from build123d import *

# Parameters (mm, degrees)
BOSS_EXTRUDE1_DEPTH      = 0.5
BOSS_EXTRUDE1_DEPTH_BACK = 38
SKETCH1_R                = 2
BOSS_EXTRUDE2_DEPTH      = 1
BOSS_EXTRUDE2_DEPTH_BACK = 0.2
FILLET1_R                = 1
SKETCH3_W                = 9.33031097
SKETCH3_H                = 7.737675748
BOSS_EXTRUDE3_DEPTH      = 0.5


with BuildPart() as part:
    # Sketch1 → Boss-Extrude1 (new, two sides: drawn at the far end of the back side and taken through both)
    with BuildSketch(Plane.XY.offset(-BOSS_EXTRUDE1_DEPTH_BACK)):
        with Locations((36.163012657, 38.866961635)):
            Circle(SKETCH1_R)
    extrude(amount=BOSS_EXTRUDE1_DEPTH + BOSS_EXTRUDE1_DEPTH_BACK)

    # Sketch2 → Boss-Extrude2 (add, two sides: drawn at the far end of the back side and taken through both)
    with BuildSketch(Plane.XY.offset(0.5).offset(-BOSS_EXTRUDE2_DEPTH_BACK)):
        with BuildLine():
            Line((36.163012657, 33.665102482), (42.084431795, 43.04323939))
            add(Edge.make_bspline(
                [(42.084431795, 43.04323939), (36.188063939, 40.196898594), (30.297901751, 43.04323939)],
                knots=[0, 0, 0, 1, 1, 1], degree=2))
            Line((30.297901751, 43.04323939), (36.163012657, 33.665102482))
        make_face()
    extrude(amount=BOSS_EXTRUDE2_DEPTH + BOSS_EXTRUDE2_DEPTH_BACK)

    # Fillet1
    fillet1_edges = [part.edges().sort_by_distance(p)[0] for p in [
        (33.230457204, 38.354170936, 1.5),
        (39.123722226, 38.354170936, 1.5),
        (36.189615356, 41.620068992, 1.5),
    ]]
    fillet(fillet1_edges, radius=FILLET1_R - 0.0001)  # a hair under: the kernel refuses the full size

    # Sketch3 → Boss-Extrude3 (add)
    with BuildSketch(Plane.XY.offset(-2.1)):
        with Locations((36.163012657, 38.866961635)):
            Rectangle(SKETCH3_W, SKETCH3_H)
    extrude(amount=-BOSS_EXTRUDE3_DEPTH)


solid = part.part
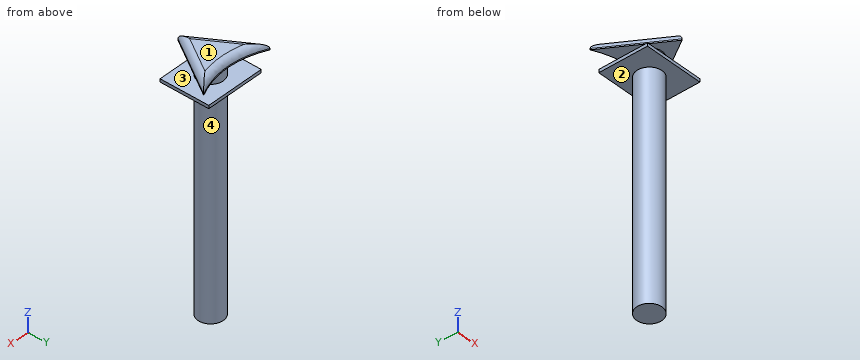
Design review of the part built by this model. Coordinates are the model's own, in mm. Face numbers are marked on the shaded views. Round coordinates to 2 decimals unless told otherwise and drop trailing zeros. Order: outer loops, then holes, each group sorted by start corner. A loop starts at its lowest first (then second) coordinate and runs counter-clockwise, first axis right, second up.
1) Clearance check with flat-ended pins moving along their axes: pin 1 Ø0.6 at (x, z) = (34.5, -2.5) entering from -Y; pin 2 Ø2.5 at (x, y) = (34, 37.5) entering from -Z; pin 3 Ø0.6 at (y, z) = (37.5, -2.5) entering from -X; pin 4 Ø1 at (y, z) = (38.5, -10.5) entering from +X. State where each tip first meets the part, or that it passes through.
The answers:
pin 1: stops at y = 35
pin 2: stops at z = -38
pin 3: stops at x = 31.5
pin 4: stops at x = 38.16
2) For L1, parallel to Z at x = 34, y = 40.5; L2, parallel to Z at x = 38.25, y = 35.5; L3, parallel to Z at x = 38, y = 41.5, list the stretches that pass through material, from the lowest coordinate up.
The answers:
L1: z = -2.6 to -2.1, 0.3 to 1.5
L2: z = -2.6 to -2.1
L3: z = -2.6 to -2.1, 0.3 to 1.16
3) Consider section A-A (y = 42.25). Count the separate pieces of the cut face and the enclosed holes in it, plus the area to 3 significant figures.
The answers:
separate pieces: 3
enclosed holes: 0
area: 6.80 mm2
4) Draft analysis for pull direction Z (two halves, no side actions). For the marked faces 1, 2, 3 and 4, state which applies: released by +Z, released by -Z, zero draft, split by the parting line, or undercut.
The answers:
face 1: released by +Z
face 2: released by -Z
face 3: undercut
face 4: zero draft
5) Consider section B-B (z = -34). State the section outline as (x, y) points.
The answers:
outline: circle Ø4 at (36.16, 38.87)
